```python
from build123d import *

# Parameters (mm, degrees)
FILLET1_R = 76.2


# Read off the part's stored shape, not the designer's step: Shell1
with BuildPart() as part:
    # Sketch1 → Revolve1 (revolve)
    with BuildSketch(Plane.XY, mode=Mode.PRIVATE) as revolve1_sk:
        Polygon((0, 308.61), (0, 0), (27.051, 0), (27.051, 95.25), (11.811, 308.61), align=None)
    revolve(revolve1_sk.sketch.rotate(Axis((0, 473.964, 0), (0, -1, 0)), 90), axis=Axis((0, 473.964, 0), (0, -1, 0)))

    # Shell1 outline → Shell1 (revolve, cut)
    with BuildSketch(Plane.XY):
        Polygon((25.4, 0), (25.4, 95.191110733), (10.155793624, 308.61), (0, 308.61), (0, 0), align=None)
    revolve(axis=Axis((0, 0, 0), (0, 1, 0)), mode=Mode.SUBTRACT)

    # Fillet1
    # the kernel refuses this fillet: 76.2 mm, written as the material it takes off along each edge
    with BuildSketch(Plane(origin=(0, 95.25, 0), x_dir=(0, 0, 1), z_dir=(1, 0, 0))) as fillet1_piece_1:
        with BuildLine():
            CenterArc((27.051 - FILLET1_R, FILLET1_R * 0.0356688476182), FILLET1_R, 355.91438322, 4.08561678)
            Line((27.051 - FILLET1_R * 0.00254130016926, -FILLET1_R * 0.0355782023697), (27.051 + FILLET1_R * 0.0174078738273, -FILLET1_R * 0.0370031433695))
            Line((27.051 + FILLET1_R * 0.0174078738273, -FILLET1_R * 0.0370031433695), (27.051 + FILLET1_R * 0.02, -FILLET1_R * 0.000713376952364))
            Line((27.051 + FILLET1_R * 0.02, -FILLET1_R * 0.000713376952364), (27.051 + FILLET1_R * 0.02, FILLET1_R * 0.0356688476182))
            Line((27.051 + FILLET1_R * 0.02, FILLET1_R * 0.0356688476182), (27.051, FILLET1_R * 0.0356688476182))
        make_face()
    revolve(axis=Axis((0, 95.25, 0), (0, -1, 0)), mode=Mode.SUBTRACT)


solid = part.part
```
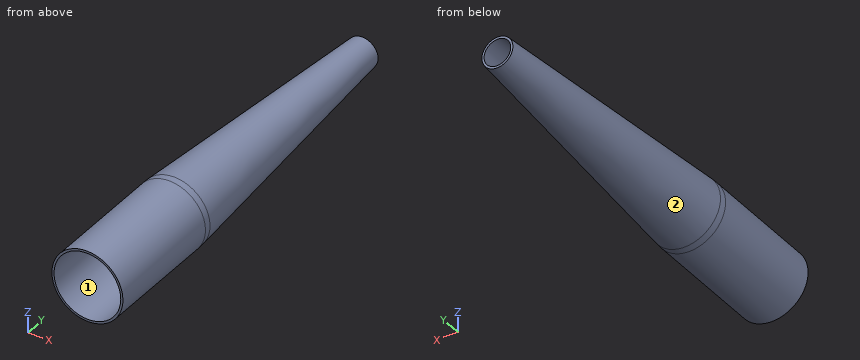
Model file for the job. Use its own axes, mm. Face numbers are marked on the shaded views. Coordinates: 2 decimals unless noted, no trailing zeros. Write each loop counter-clockwise with the first axis right and the second up, starting at its lowest first coordinate (ties: lowest second). Pieces come first, ordered by that corner, then holes. Notation, with made-up numbers: (-19, -32.5) - (32, -32.5) arc R23 ccw to (32, -11.5) - close; hole circle Ø11 at (6.25, 16.25). An arc over 180 degrees is marked (long way). One line per question, with ' | ' between items. Start each with the question number.
Q1. Cut at A-A, the plane y = 66. List the corners of the cut face in (x, z).
Q2. Drill centre lines: line 1 (X direction, y = 28, z = 0); line 2 (Z direction, x = -0.5, y = 132.5). Where is each one in solid material? Low to high. Write a range as [from, to].
Q3. Pin check, flat tips, straight feed: pin 1 (1.5 mm diameter, centred on y = 99, z = 20.5, fed in from +X); pin 2 (1.5 mm diameter, centred on y = 261.5, z = -8.5, fed in from +X); pin 3 (10 mm diameter, centred on x = 9.5, z = 9, fed in from +Y); pin 4 (2 mm diameter, centred on y = 50.5, z = 8, fed in from +X). Stop position of each tip, or through.
Q4. Cut at B-B, the plane y = 206. List the corners of the cut face in (x, z).
Q5. Pull direction Z, two halves, no side cores. Call the marked faces 1 and 2: pulls with the +Z half, pulls with the -Z half, needs draft (parallel to the pull), parting line crosses it, or undercut.
Answer below:
1) outline: circle Ø54.1 at (0, 0); hole circle Ø50.8 at (0, 0)
2) line 1: [-27.05, -25.4], [25.4, 27.05] | line 2: [-24.39, -22.73], [22.73, 24.39]
3) pin 1: x = 18.09 | pin 2: x = 13.05 | pin 3: y = 308.61 | pin 4: x = 26.13
4) outline: circle Ø38.28 at (0, 0); hole circle Ø34.97 at (0, 0)
5) face 1: undercut | face 2: parting line crosses it
